from build123d import *

# Parameters (mm, degrees)
F0_R     = 1.5
F1_DEPTH = 10
F3_R     = 1.5
F4_DEPTH = 10
F5_DEPTH = 2


with BuildPart() as f1:
    # F0 (on Front) → F1 (new body)
    with BuildSketch(Plane.XZ):
        Circle(F0_R)
    extrude(amount=-F1_DEPTH)



with BuildPart() as f4:
    # F3 (on Front) → F4 (new body, through all)
    with BuildSketch(Plane.XZ):
        with Locations((0, -40)):
            Circle(F3_R)
    extrude(amount=-F4_DEPTH)


with BuildPart() as f1_1:
    add(f1.part)

    add(f4.part)  # F5 merges F4
    # F2 (on Front) → F5 (join)
    with BuildSketch(Plane.XZ):
        with BuildLine():
            ThreePointArc((3, 0), (0, 3), (-3, 0))
            Line((-3, 0), (-3, -40))
            ThreePointArc((-3, -40), (0, -43), (3, -40))
            Line((3, -40), (3, 0))
        make_face()
    extrude(amount=-F5_DEPTH)


solid = f1_1.part
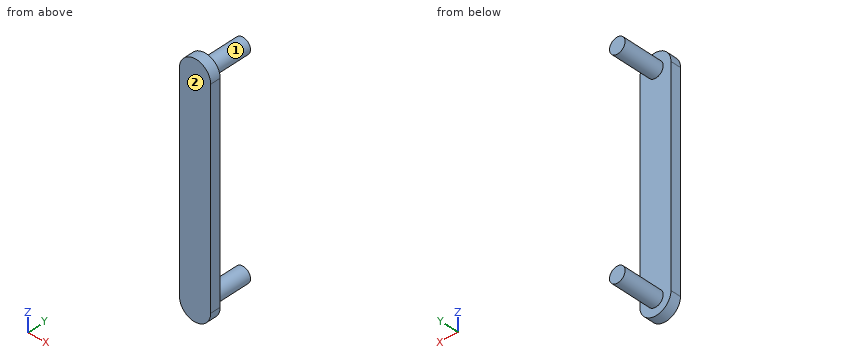
Can you work these out from the model? Positions are in its coordinate system, mm. Face numbers are marked on the shaded views. Give positions to 0.01 mm unless a question says otherwise; leave off trailing zeros. Loops run counter-clockwise (first coordinate to the right, second up) from the corner with the lowest first, then second, coordinate; pieces in that order, holes last. Notation, with made-up numbers: (51.5, 83.25) - (81.5, 83.25) arc R14 cw to (81.5, 87.25) - close; hole circle Ø3 at (84.25, -39). An arc over 180 degrees is marked (long way). One line per item, written item: value.
(1) I need wall thicknesses on line 1 along Y through (x, z) = (1.85, -9.5); line 2 along Z through (x, y) = (-0.25, 2.25); line 3 along Z through (x, y) = (0.2, 1.25). Which ranges of each line are inside material? Lowest first, please.
Verdict:
line 1: 0 to 2
line 2: -41.48 to -38.52, -1.48 to 1.48
line 3: -42.99 to 2.99
(2) If we mould it in two halves opening along Z, with no side actions, what happens to the marked faces 1 and 2? For each: released by +Z, released by -Z, zero draft, split by the parting line, or undercut.
Verdict:
face 1: undercut
face 2: zero draft
(3) If we section it at C-C, the plane z = -9.5: List the corners of the cut face in (x, y) for me.
Verdict:
outline: (-3, 0) - (3, 0) - (3, 2) - (-3, 2) - close
(4) If we section it at B-B, the plane x = 0: List the corners of the cut face in (y, z) for me, plus the area to 3 significant figures.
Verdict:
outline: (0, -43) - (2, -43) - (2, -41.5) - (10, -41.5) - (10, -38.5) - (2, -38.5) - (2, -1.5) - (10, -1.5) - (10, 1.5) - (2, 1.5) - (2, 3) - (0, 3) - close
area: 140 mm^2
(5) If we section it at A-A, the plane y = 4: List the corners of the cut face in (x, z) for me, plus the area to 3 significant figures.
Verdict:
outline: circle Ø3 at (0, -40); circle Ø3 at (0, 0)
area: 14.1 mm^2
(6) I'm going to push flat-ended pins straight in: pin 1 (3 mm diameter, centred on x = 0, z = -7.5, fed in from +Y); pin 2 (2 mm diameter, centred on y = 4.5, z = -23, fed in from +X). Where does each tip first touch, or does it pass through?
Verdict:
pin 1: y = 2
pin 2: through
(7) If we section it at D-D, the plane y = 1.5: List the corners of the cut face in (x, z) for me.
Verdict:
outline: (-3, -40) arc R3 ccw to (3, -40) - (3, 0) arc R3 ccw to (-3, 0) - close
